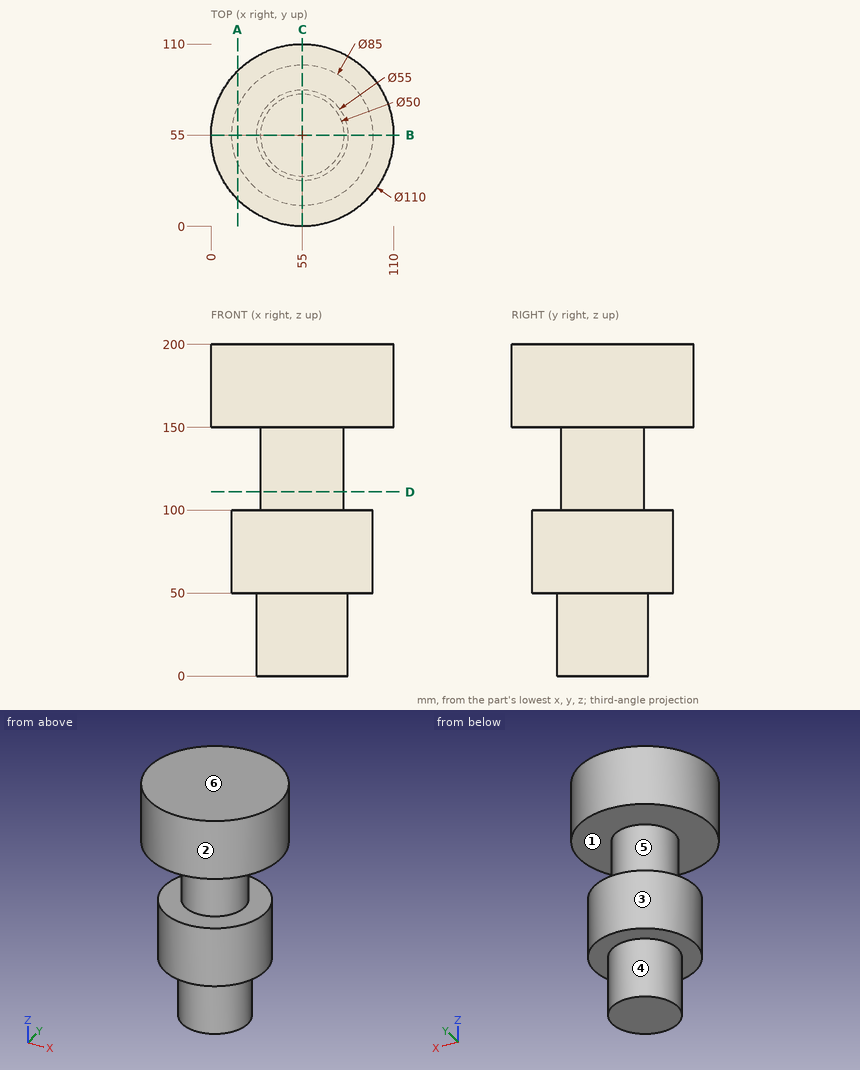
Job drawing, mm, ordinate dimensions from the low corner. One solid piece. A direction names the side the tool comes from. Round coordinates to 2 decimals unless told otherwise and drop trailing zeros. Loops run counter-clockwise (first coordinate to the right, second up) from the corner with the lowest first, then second, coordinate; pieces in that order, holes last.
(1) Which spindle directions (+Z, -Z, +X, -X, +Y, -Y) get a long thin tool onto all of the face, cutting with end or side? Do the marked faces 1, 2 and 3. Say none if no direction does.
(2) Wall check: line 1 along Z through (x, y) = (91.5, 74.5); line 2 along Z through (x, y) = (96, 20.5); line 3 along Y through (x, z) = (59.5, 130). Give the ranges that are in metal, low to high.
(3) Cut at A-A (x = 16). Give the cut face in (y, z), plus the area to 3 significant figures.
(4) Drop flat-ended pins along their axis: pin 1 (8 mm diameter, centred on x = 19.5, y = 77.5, fed in from -Z); pin 2 (2 mm diameter, centred on x = 51.5, z = 69.5, fed in from -Y); pin 3 (2 mm diameter, centred on y = 22, z = 168, fed in from +X); pin 4 (10 mm diameter, centred on x = 62, y = 36.5, fed in from -Z). Give the stop position or say it passes through.
(5) Cut at B-B (y = 55). Give the cut face in (x, z), plus the area to 3 significant figures.
(6) Two-plate mould, pull along Z, no slides. Class the marked faces 4, 5 and 6: +Z half, -Z half, draft (parallel to the pull), parting line (faces both ways), or undercut.
(7) Cut at D-D (z = 111). Give the cut face in (x, y).
Findings below:
1. face 1: none
1. face 2: +Z, -Z
1. face 3: -Z
2. line 1: z = 50 to 100, 150 to 200
2. line 2: z = 150 to 200
2. line 3: y = 30.41 to 79.59
3. outline: (16.22, 150) - (93.78, 150) - (93.78, 200) - (16.22, 200) - close; (38.11, 50) - (71.89, 50) - (71.89, 100) - (38.11, 100) - close
3. area: 5,570 mm2
4. pin 1: stops at z = 50
4. pin 2: stops at y = 12.57
4. pin 3: stops at x = 99.73
4. pin 4: stops at z = 0
5. outline: (0, 150) - (30, 150) - (30, 100) - (12.5, 100) - (12.5, 50) - (27.5, 50) - (27.5, 0) - (82.5, 0) - (82.5, 50) - (97.5, 50) - (97.5, 100) - (80, 100) - (80, 150) - (110, 150) - (110, 200) - (0, 200) - close
5. area: 15,000 mm2
6. face 4: draft
6. face 5: undercut
6. face 6: +Z half
7. outline: circle Ø50 at (55, 55)
